Source: CAD feature listing. Evaluate the final solid. Frame: model axes, mm. Face numbers are marked on the shaded views. Coordinates: 2 decimals unless noted, no trailing zeros. Order: outer loops, then holes, each group sorted by start corner. A loop starts at its lowest first (then second) coordinate and runs counter-clockwise, first axis right, second up. Notation, with made-up numbers: (78.5, 63.25) -> (117.5, 63.25) arc R24 ccw to (117.5, 95.25) -> close; hole circle Ø6 at (84.25, 56). An arc over 180 degrees is marked (long way). Write each question's results on one line, items separated by ' | '. Start each with the question number.
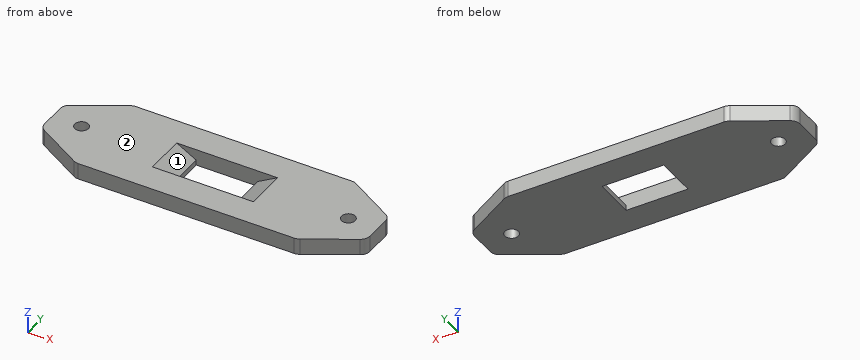
from build123d import *

# Parameters (mm, degrees)
SKETCH1_W             = 100
SKETCH1_H             = 30
BOSS_EXTRUDE1_DEPTH   = 5
CHAMFER1_SIZE         = 16
CHAMFER1_SIZE2        = 9.237604307
CHAMFER1_PART_2_SIZE  = 16
CHAMFER1_PART_2_SIZE2 = 9.237604307
FILLET1_R             = 3
SKETCH2_R             = 2.1
CUT_EXTRUDE1_DEPTH    = 6
SKETCH3_W             = 19
SKETCH3_H             = 12.6
CUT_EXTRUDE2_DEPTH    = 6
CHAMFER2_SIZE         = 6
CHAMFER2_SIZE2        = 3.4


with BuildPart() as part:
    # Sketch1 → Boss-Extrude1 (new body)
    with BuildSketch(Plane.XY):
        with Locations((-50, 15)):
            Rectangle(SKETCH1_W, SKETCH1_H)
    extrude(amount=BOSS_EXTRUDE1_DEPTH)

    # Chamfer1
    chamfer1_edges = [part.edges().sort_by_distance(p)[0] for p in [
        (0, 0, 2.5),
        (-100, 0, 2.5),
    ]]
    chamfer1_side = [part.faces().sort_by_distance(p)[0] for p in [
        (-50, 0, 2.5),
    ]]
    chamfer(chamfer1_edges, length=CHAMFER1_SIZE, length2=CHAMFER1_SIZE2, reference=chamfer1_side[0])

    # Chamfer1 part 2
    chamfer1_part_2_edges = [part.edges().sort_by_distance(p)[0] for p in [
        (-100, 30, 2.5),
        (0, 30, 2.5),
    ]]
    chamfer1_part_2_side = [part.faces().sort_by_distance(p)[0] for p in [
        (-50, 30, 2.5),
    ]]
    chamfer(chamfer1_part_2_edges, length=CHAMFER1_PART_2_SIZE, length2=CHAMFER1_PART_2_SIZE2, reference=chamfer1_part_2_side[0])

    # Fillet1
    fillet1_edges = [part.edges().sort_by_distance(p)[0] for p in [
        (-84, 30, 2.5),
        (-16, 30, 2.5),
        (0, 9.237604307, 2.5),
        (0, 20.762395693, 2.5),
        (-84, 0, 2.5),
        (-16, 0, 2.5),
        (-100, 20.762395693, 2.5),
        (-100, 9.237604307, 2.5),
    ]]
    fillet(fillet1_edges, radius=FILLET1_R)

    # Sketch2 → Cut-Extrude1 (cut, through all)
    with BuildSketch(Plane.XY.offset(5)):
        with Locations((-91, 15)):
            Circle(SKETCH2_R)
        with Locations((-9, 15)):
            Circle(SKETCH2_R)
    extrude(amount=-CUT_EXTRUDE1_DEPTH, mode=Mode.SUBTRACT)

    # Sketch3 → Cut-Extrude2 (cut, through all)
    with BuildSketch(Plane.XY.offset(5)):
        with Locations((-50, 15)):
            Rectangle(SKETCH3_W, SKETCH3_H)
    extrude(amount=-CUT_EXTRUDE2_DEPTH, mode=Mode.SUBTRACT)

    # Chamfer2
    chamfer2_edges = [part.edges().sort_by_distance(p)[0] for p in [
        (-59.5, 15, 5),
        (-40.5, 15, 5),
    ]]
    chamfer2_side = [part.faces().sort_by_distance(p)[0] for p in [
        (-1.044030651, 15, 5),
    ]]
    chamfer(chamfer2_edges, length=CHAMFER2_SIZE, length2=CHAMFER2_SIZE2, reference=chamfer2_side[0])


solid = part.part
(1) Section B-B on z = 2.45. Return the cut outline in (x, y).
(2) Line query: L1, parallel to Y at x = -59, z = 2.25; L2, parallel to Y at x = -9, z = 3.5; L3, parallel to X at y = 21, z = 4.45. Output: solid intervals per line, ascending.
(3) Section C-C on y = 15. Return the cut outline in (x, z).
(4) Draft query along X for the marked faces 1 and 2. Return one class per face: released by +X, released by -X, zero draft, split by the parting line, or undercut.
(5) Section D-D on x = -91. Return the cut outline in (y, z), then the cut area to 3 significant figures.
(6) First-contact query: P1, Ø1, axis at y = 24, z = 1, coming from the +X side. Flat tip, straight axial feed; report the tip coordinate or a pass-through.
(7) Section A-A on x = -52. Return the cut outline in (y, z), then the cut area to 3 significant figures.
Results list:
1) outline: (-100, 10.97) arc R3 ccw to (-98.5, 8.37) -> (-84.7, 0.4) arc R3 ccw to (-83.2, 0) -> (-16.8, 0) arc R3 ccw to (-15.3, 0.4) -> (-1.5, 8.37) arc R3 ccw to (0, 10.97) -> (0, 19.03) arc R3 ccw to (-1.5, 21.63) -> (-15.3, 29.6) arc R3 ccw to (-16.8, 30) -> (-83.2, 30) arc R3 ccw to (-84.7, 29.6) -> (-98.5, 21.63) arc R3 ccw to (-100, 19.03) -> close; hole circle Ø4.2 at (-91, 15); hole (-61, 8.7) -> (-39, 8.7) -> (-39, 21.3) -> (-61, 21.3) -> close; hole circle Ø4.2 at (-9, 15)
2) L1: y = 0 to 8.7, 21.3 to 30 | L2: y = 4.04 to 12.9, 17.1 to 25.96 | L3: x = -99.26 to -64.53, -35.47 to -0.74
3) outline: (-100, 0) -> (-93.1, 0) -> (-93.1, 5) -> (-100, 5) -> close; (-88.9, 0) -> (-59.5, 0) -> (-59.5, 1.6) -> (-65.5, 5) -> (-88.9, 5) -> close; (-40.5, 0) -> (-11.1, 0) -> (-11.1, 5) -> (-34.5, 5) -> (-40.5, 1.6) -> close; (-6.9, 0) -> (0, 0) -> (0, 5) -> (-6.9, 5) -> close
4) face 1: undercut | face 2: zero draft
5) outline: (4.04, 0) -> (12.9, 0) -> (12.9, 5) -> (4.04, 5) -> close; (17.1, 0) -> (25.96, 0) -> (25.96, 5) -> (17.1, 5) -> close | area: 88.6 mm²
6) P1: stops at x = -4.74
7) outline: (0, 0) -> (8.7, 0) -> (8.7, 5) -> (0, 5) -> close; (21.3, 0) -> (30, 0) -> (30, 5) -> (21.3, 5) -> close | area: 87.0 mm²
